```python
from build123d import *

# Parameters (mm, degrees)
F1_DEPTH       = 2
F2_DEPTH       = 25
F3_R           = 2
F4_T1_DEPTH    = 29
F4_T3_DEPTH    = 29
F4_T5_DEPTH    = 29
F4_T7_DEPTH    = 29
F4_T9_DEPTH    = 43.2
F4_T11_DEPTH   = 43.2
F5_R           = 2
F6_SIZE        = 2
F8_D           = 3.3
F8_CSINK_D     = 6
F8_CSINK_ANGLE = 90


# Not quite as in the source:
# - a fillet or chamfer that OpenCascade refuses, or shapes differently, is made with other operations: its cross-section is extruded or revolved along the edge and cut away or added


with BuildPart() as f1:
    # F0 (on Top) → F1 (new body)
    with BuildSketch(Plane.XY):
        Polygon((-28.4735770881, 0), (0, 0), (28.4735770881, 0), (28.4735770881, 10.2), (5.1, 10.2), (5.1, 33.5735770881), (-5.1, 33.5735770881), (-5.1, 10.2), (-28.4735770881, 10.2), align=None)
        Polygon((28.4735770881, 0), (0, 0), (-28.4735770881, 0), (-28.4735770881, -4), (0, -4), (28.4735770881, -4), align=None)
        Polygon((5.1, 10.2), (28.4735770881, 10.2), (28.4735770881, 14.2), (9.1, 14.2), (9.1, 33.5735770881), (5.1, 33.5735770881), align=None)
        Polygon((-28.4735770881, 14.2), (-28.4735770881, 10.2), (-5.1, 10.2), (-5.1, 33.5735770881), (-9.1, 33.5735770881), (-9.1, 14.2), align=None)
    extrude(amount=F1_DEPTH)

    # F0 (on Top) → F2 (join)
    with BuildSketch(Plane.XY):
        Polygon((-28.4735770881, 14.2), (-28.4735770881, 10.2), (-5.1, 10.2), (-5.1, 33.5735770881), (-9.1, 33.5735770881), (-9.1, 14.2), align=None)
        Polygon((5.1, 10.2), (28.4735770881, 10.2), (28.4735770881, 14.2), (9.1, 14.2), (9.1, 33.5735770881), (5.1, 33.5735770881), align=None)
        Polygon((28.4735770881, 0), (0, 0), (-28.4735770881, 0), (-28.4735770881, -4), (0, -4), (28.4735770881, -4), align=None)
    extrude(amount=F2_DEPTH)

    # F3
    f3_edges = [f1.edges().sort_by_distance(p)[0] for p in [
        (9.1, 14.2, 12.5),
    ]]
    fillet(f3_edges, radius=F3_R)

    # F4: fillet of radius 5 on 9 edges, made by hand

    # F4_s2 → F4_t1 (cut)
    with BuildSketch(Plane.XZ.offset(-12.5)):
        with BuildLine():
            ThreePointArc((28.4735770881, 20), (27.0091109941, 23.5355339059), (23.4735770881, 25))
            Line((23.4735770881, 25), (28.4735770881, 25))
            Line((28.4735770881, 25), (28.4735770881, 20))
        make_face()
        with BuildLine():
            ThreePointArc((-28.4735770881, 20), (-27.0091109941, 23.5355339059), (-23.4735770881, 25))
            Line((-23.4735770881, 25), (-28.4735770881, 25))
            Line((-28.4735770881, 25), (-28.4735770881, 20))
        make_face()
    extrude(amount=F4_T1_DEPTH, mode=Mode.SUBTRACT)

    # F4_s4 → F4_t3 (cut)
    with BuildSketch(Plane.XZ.offset(-26.7)):
        with BuildLine():
            ThreePointArc((28.4735770881, 20), (27.0091109941, 23.5355339059), (23.4735770881, 25))
            Line((23.4735770881, 25), (28.4735770881, 25))
            Line((28.4735770881, 25), (28.4735770881, 20))
        make_face()
        with BuildLine():
            ThreePointArc((-28.4735770881, 20), (-27.0091109941, 23.5355339059), (-23.4735770881, 25))
            Line((-23.4735770881, 25), (-28.4735770881, 25))
            Line((-28.4735770881, 25), (-28.4735770881, 20))
        make_face()
    extrude(amount=F4_T3_DEPTH, mode=Mode.SUBTRACT)

    # F4_s6 → F4_t5 (cut)
    with BuildSketch(Plane.YZ.offset(-21.6)):
        with BuildLine():
            ThreePointArc((33.5735770881, 20), (32.1091109941, 23.5355339059), (28.5735770881, 25))
            Line((28.5735770881, 25), (33.5735770881, 25))
            Line((33.5735770881, 25), (33.5735770881, 20))
        make_face()
    extrude(amount=F4_T5_DEPTH, mode=Mode.SUBTRACT)

    # F4_s8 → F4_t7 (cut)
    with BuildSketch(Plane.YZ.offset(-7.4)):
        with BuildLine():
            ThreePointArc((33.5735770881, 20), (32.1091109941, 23.5355339059), (28.5735770881, 25))
            Line((28.5735770881, 25), (33.5735770881, 25))
            Line((33.5735770881, 25), (33.5735770881, 20))
        make_face()
    extrude(amount=F4_T7_DEPTH, mode=Mode.SUBTRACT)

    # F4_s10 → F4_t9 (cut)
    with BuildSketch(Plane.XZ.offset(-26.7)):
        with BuildLine():
            ThreePointArc((-23.4735770881, 0), (-27.0091109941, 1.4644660941), (-28.4735770881, 5))
            Line((-28.4735770881, 5), (-28.4735770881, 0))
            Line((-28.4735770881, 0), (-23.4735770881, 0))
        make_face()
        with BuildLine():
            ThreePointArc((23.4735770881, 0), (27.0091109941, 1.4644660941), (28.4735770881, 5))
            Line((28.4735770881, 5), (28.4735770881, 0))
            Line((28.4735770881, 0), (23.4735770881, 0))
        make_face()
    extrude(amount=F4_T9_DEPTH, mode=Mode.SUBTRACT)

    # F4_s12 → F4_t11 (cut)
    with BuildSketch(Plane.YZ.offset(-21.6)):
        with BuildLine():
            ThreePointArc((28.5735770881, 0), (32.1091109941, 1.4644660941), (33.5735770881, 5))
            Line((33.5735770881, 5), (33.5735770881, 0))
            Line((33.5735770881, 0), (28.5735770881, 0))
        make_face()
    extrude(amount=F4_T11_DEPTH, mode=Mode.SUBTRACT)

    # F5
    f5_edges = [f1.edges().sort_by_distance(p)[0] for p in [
        (-9.1, 14.2, 12.5),
    ]]
    fillet(f5_edges, radius=F5_R)

    # F6
    f6_edges = [f1.edges().sort_by_distance(p)[0] for p in [
        (5.1, 10.2, 13.5),
        (-5.1, 10.2, 13.5),
    ]]
    chamfer(f6_edges, length=F6_SIZE)

    # F8 (through all)
    with Locations(Plane(origin=(0, 0, 0), x_dir=(1, 0, 0), z_dir=(0, 0, -1))):
        with Locations((-15, -5.1), (0, -20.1), (15, -5.1)):
            CounterSinkHole(F8_D / 2, F8_CSINK_D / 2, counter_sink_angle=F8_CSINK_ANGLE)


solid = f1.part
```
Here's how the part is built. I have some questions about the finished solid (model axes, mm). A direction names the side the tool comes from. Give positions to 0.01 mm unless a question says otherwise; leave off trailing zeros. Order: outer loops, then holes, each group sorted by start corner. A loop starts at its lowest first (then second) coordinate and runs counter-clockwise, first axis right, second up. Notation, with made-up numbers: M 4.5,7 L 37.5,7 A18 ccw 37.5,18 Z; hole C -28,34 d3. An arc over 180 degrees is marked long. Use a Markdown table: item, result. Add a question column.
1. On a 3-axis mill with a long thin cutter (end or side, diameter ignored), from which of +Z, -Z, +X, -X, +Y, -Y can I reach the whole of each face in a straight line? I mean faces 1 (the flat face through (-6.1, 11.2, 13.3)), 2 (the conical face through (13, 5, 1)), 3 (the flat face through (5.1, 23, 13)). Say none if no direction works.
2. Suppose I cut it at B-B (y = 20.1). List the corners of the cut face in (x, z) for me, and give its area (3 significant figures).
3. If we mould it in two halves opening along X, with no side actions, what happens to faces 4 (the cylindrical face through (9.7, 14.77, 12.32)), 5 (the flat face through (18, 10.2, 13)), 6 (the conical face through (-2, 20, 1)), 7 (the conical face through (-17, 5, 1))? For each: +X half, -X half, draft (parallel to the pull), parting line (faces both ways), or undercut.
4. For pin 1 Ø12 at (x, z) = (-21, 12.5) entering from +Y; pin 2 Ø8.5 at (y, z) = (28.5, 9) entering from -X; pin 3 Ø5.5 at (x, y) = (15, 5.1) entering from -Z, each with a flat end and sliding along its axis, tell me the tip position at first contact or that it passes through.
5. Suppose I cut it at C-C (x = 0). List the corners of the cut face in (y, z) for me.
6. I need wall thicknesses on probe 1 along X at (y, z) = (20.1, 1.75); probe 2 along X at (y, z) = (24, 21.5); probe 3 along Y at (x, z) = (12, 18). Which ranges of each line are inside material? Lowest first, please. Write a range as from..to.
7. Suppose I cut it at D-D (y = 5.1). List the corners of the cut face in (x, z) for me, and give its area (3 significant figures).
8. Suppose I cut it at A-A (z = 8.5). List the corners of the cut face in (x, y) for me, and give its area (3 significant figures).
Results list:
| question | item | result |
|---|---|---|
| 1 | face 1 | +Z |
| 1 | face 2 | -Z |
| 1 | face 3 | +Z, +Y |
| 2 | outline | M -9.1,0 L -3,0 L -1.65,1.35 L -1.65,2 L -5.1,2 L -5.1,25 L -9.1,25 Z; M 1.65,1.35 L 3,0 L 9.1,0 L 9.1,25 L 5.1,25 L 5.1,2 L 1.65,2 Z |
| 2 | area | 212 mm² |
| 3 | face 4 | +X half |
| 3 | face 5 | draft |
| 3 | face 6 | undercut |
| 3 | face 7 | undercut |
| 4 | pin 1 | stops at y = 14.2 |
| 4 | pin 2 | stops at x = -9.1 |
| 4 | pin 3 | stops at z = 0.25 |
| 5 | outline | M -4,0 L 17.1,0 L 18.45,1.35 L 18.45,2 L 0,2 L 0,25 L -4,25 Z; M 21.75,1.35 L 23.1,0 L 28.57,0 A5 ccw 32.57,2 L 21.75,2 Z |
| 6 | probe 1 | x = -9.1..-1.65, 1.65..9.1 |
| 6 | probe 2 | x = -9.1..-5.1, 5.1..9.1 |
| 6 | probe 3 | y = -4..0, 10.2..14.2 |
| 7 | outline | M -27.47,2 A5 ccw -23.47,0 L -18,0 L -16.65,1.35 L -16.65,2 Z; M -13.35,1.35 L -12,0 L 12,0 L 13.35,1.35 L 13.35,2 L -13.35,2 Z; M 16.65,1.35 L 18,0 L 23.47,0 A5 ccw 27.47,2 L 16.65,2 Z |
| 7 | area | 88.2 mm² |
| 8 | outline | M -28.47,-4 L 28.47,-4 L 28.47,0 L -28.47,0 Z; M -28.47,10.2 L -7.1,10.2 L -5.1,12.2 L -5.1,33.57 L -9.1,33.57 L -9.1,16.2 A2 cw -11.1,14.2 L -28.47,14.2 Z; M 5.1,12.2 L 7.1,10.2 L 28.47,10.2 L 28.47,14.2 L 11.1,14.2 A2 cw 9.1,16.2 L 9.1,33.57 L 5.1,33.57 Z |
| 8 | area | 567 mm² |
